Read the model definition and answer for the solid it produces. Units are mm, in the model's axes. A direction names the side the tool comes from. Coordinates: 2 decimals unless noted, no trailing zeros. Write each loop counter-clockwise with the first axis right and the second up, starting at its lowest first coordinate (ties: lowest second). Pieces come first, ordered by that corner, then holes. Notation, with made-up numbers: (86, 77.25) -> (132, 77.25) arc R29 ccw to (132, 101.25) -> close; hole circle Ø9 at (-40, -20.75). An arc over 180 degrees is marked (long way). Return JSON: item names as keys, results as strings.
from build123d import *

# Parameters (mm, degrees)
F1_W     = 740
F1_H     = 640
F1_W_2   = 20
F1_H_2   = 600
F2_DEPTH = 20
F0_R     = 1.4
F0_R_2   = 1.9
F0_W     = 5
F0_H     = 5
F0_R_3   = 16
F3_DEPTH = 5
F4_W     = 20
F4_H     = 20
F5_DEPTH = 700


with BuildPart() as f2:
    # F1 (on Top) → F2 (new body)
    with BuildSketch(Plane.XY):
        with Locations((0, -40)):
            Rectangle(F1_W, F1_H)
        Polygon((-350, -340), (-350, 260), (-147.5, 260), (-127.5, 260), (127.5, 260), (147.5, 260), (350, 260), (350, -340), (147.5, -340), (127.5, -340), (-127.5, -340), (-147.5, -340), align=None, mode=Mode.SUBTRACT)
        with Locations((137.5, -40)):
            Rectangle(F1_W_2, F1_H_2)
        with Locations((-137.5, -40)):
            Rectangle(F1_W_2, F1_H_2)
    extrude(amount=-F2_DEPTH)

    # F0 (on Top) → F3 (join)
    with BuildSketch(Plane.XY):
        with BuildLine():
            Line((330, -340), (-330, -340))
            Line((-330, -340), (-330, -379.616912))
            ThreePointArc((-330, -379.616912), (0, -503), (330, -379.616912))
            Line((330, -379.616912), (330, -340))
        make_face()
        with Locations((-285.202138, -385.913671)):
            Circle(F0_R, mode=Mode.SUBTRACT)
        with Locations((-313.348072, -363.468038)):
            Circle(F0_R, mode=Mode.SUBTRACT)
        with Locations((-124.358751, -463.371764)):
            Circle(F0_R, mode=Mode.SUBTRACT)
        with Locations((-89.261346, -471.382518)):
            Circle(F0_R, mode=Mode.SUBTRACT)
        with Locations((89.261346, -471.382518)):
            Circle(F0_R, mode=Mode.SUBTRACT)
        with Locations((124.358751, -463.371764)):
            Circle(F0_R, mode=Mode.SUBTRACT)
        with Locations((285.202138, -385.913671)):
            Circle(F0_R, mode=Mode.SUBTRACT)
        with Locations((313.348072, -363.468038)):
            Circle(F0_R, mode=Mode.SUBTRACT)
        with BuildLine():
            Line((330, 260), (330, 368.951685))
            Line((330, 368.951685), (330, 379.616912))
            ThreePointArc((330, 379.616912), (319.49595, 388.498826), (308.752952, 397.090185))
            Line((308.752952, 397.090185), (275.202138, 397.090185))
            Line((275.202138, 397.090185), (206.772293, 298.352508))
            ThreePointArc((206.772293, 298.352508), (146.302539, 332.21163), (80.5, 353.961509))
            Line((80.5, 353.961509), (79.396479, 349.085021))
            Line((79.396479, 349.085021), (77.189345, 339.331634))
            Line((77.189345, 339.331634), (70.567941, 310.071473))
            Line((70.567941, 310.071473), (68.360806, 300.318086))
            Line((68.360806, 300.318086), (67.03647, 294.465807))
            Line((67.03647, 294.465807), (-67.03647, 294.465807))
            Line((-67.03647, 294.465807), (-68.360806, 300.318086))
            Line((-68.360806, 300.318086), (-70.567941, 310.071473))
            Line((-70.567941, 310.071473), (-77.189345, 339.331634))
            Line((-77.189345, 339.331634), (-79.396479, 349.085021))
            Line((-79.396479, 349.085021), (-80.5, 353.961509))
            ThreePointArc((-80.5, 353.961509), (-146.302539, 332.21163), (-206.772293, 298.352508))
            Line((-206.772293, 298.352508), (-275.202138, 397.090185))
            Line((-275.202138, 397.090185), (-308.752952, 397.090185))
            ThreePointArc((-308.752952, 397.090185), (-319.49595, 388.498826), (-330, 379.616912))
            Line((-330, 379.616912), (-330, 260))
            Line((-330, 260), (330, 260))
        make_face()
        with Locations((-313.348072, 364.644552)):
            Circle(F0_R, mode=Mode.SUBTRACT)
        with Locations((-285.202138, 387.090185)):
            Circle(F0_R, mode=Mode.SUBTRACT)
        with Locations((313.348072, 364.644552)):
            Circle(F0_R, mode=Mode.SUBTRACT)
        with Locations((285.202138, 387.090185)):
            Circle(F0_R, mode=Mode.SUBTRACT)
        Polygon((77.189345, 339.331634), (79.396479, 349.085021), (74.519786, 350.188588), (72.312651, 340.435201), align=None)
        Polygon((-74.519786, 350.188588), (-79.396479, 349.085021), (-77.189345, 339.331634), (-72.312651, 340.435201), align=None)
        Polygon((68.360806, 300.318086), (70.567941, 310.071473), (65.691247, 311.17504), (63.484113, 301.421653), align=None)
        Polygon((-65.691247, 311.17504), (-70.567941, 310.071473), (-68.360806, 300.318086), (-63.484113, 301.421653), align=None)
        with BuildLine():
            Line((442.050902, 240), (350, 240))
            Line((350, 240), (350, -240))
            Line((350, -240), (442.050902, -240))
            ThreePointArc((442.050902, -240), (502.730809, -16.453988), (456.79808, 210.581372))
            Line((456.79808, 210.581372), (407.539006, 186.859452))
            Line((407.539006, 186.859452), (403.634053, 194.968172))
            Line((403.634053, 194.968172), (399.729099, 203.076892))
            Line((399.729099, 203.076892), (448.971082, 226.790581))
            ThreePointArc((448.971082, 226.790581), (445.559947, 233.420937), (442.050902, 240))
        make_face()
        with Locations((424.655149, -223.893378)):
            Circle(F0_R, mode=Mode.SUBTRACT)
        with Locations((440.274964, -191.458498)):
            Circle(F0_R, mode=Mode.SUBTRACT)
        with Locations((480, -17.411743)):
            Circle(F0_R, mode=Mode.SUBTRACT)
        with Locations((480, 18.588257)):
            Circle(F0_R, mode=Mode.SUBTRACT)
        with Locations((419.869226, 188.912666)):
            Circle(F0_R_2, mode=Mode.SUBTRACT)
        with Locations((409.022132, 211.436888)):
            Circle(F0_R_2, mode=Mode.SUBTRACT)
        with BuildLine():
            Line((-350, -240), (-350, 240))
            Line((-350, 240), (-442.050902, 240))
            ThreePointArc((-442.050902, 240), (-503, 0), (-442.050902, -240))
            Line((-442.050902, -240), (-350, -240))
        make_face()
        with Locations((-424.655149, -223.893378)):
            Circle(F0_R, mode=Mode.SUBTRACT)
        with Locations((-440.274964, -191.458498)):
            Circle(F0_R, mode=Mode.SUBTRACT)
        with Locations((-480, -17.411743)):
            Circle(F0_R, mode=Mode.SUBTRACT)
        with Locations((-480, 18.588257)):
            Circle(F0_R, mode=Mode.SUBTRACT)
        with Locations((-440.274964, 192.635012)):
            Circle(F0_R, mode=Mode.SUBTRACT)
        with Locations((-424.655149, 225.069891)):
            Circle(F0_R, mode=Mode.SUBTRACT)
        with BuildLine():
            Line((-140, 130), (-150, 130))
            Line((-150, 130), (-150, -130))
            Line((-150, -130), (-140, -130))
            Line((-140, -130), (-140, -120))
            ThreePointArc((-140, -120), (-137.5, -117.5), (-135, -120))
            Line((-135, -120), (-134.791644, -130))
            Line((-134.791644, -130), (135, -130))
            Line((135, -130), (135, -120))
            ThreePointArc((135, -120), (137.5, -117.5), (140, -120))
            Line((140, -120), (140, -130))
            Line((140, -130), (150, -130))
            Line((150, -130), (150, 130))
            Line((150, 130), (140, 130))
            Line((140, 130), (140, 120))
            ThreePointArc((140, 120), (137.5, 117.5), (135, 120))
            Line((135, 120), (135, 130))
            Line((135, 130), (-135, 130))
            Line((-135, 130), (-135, 120))
            ThreePointArc((-135, 120), (-137.5, 117.5), (-140, 120))
            Line((-140, 120), (-140, 130))
        make_face()
        with Locations((-93.691649, -118.440386)):
            Circle(F0_R, mode=Mode.SUBTRACT)
        with Locations((-118.440386, -93.691649)):
            Circle(F0_R, mode=Mode.SUBTRACT)
        with Locations((93.691649, -118.440386)):
            Circle(F0_R, mode=Mode.SUBTRACT)
        with Locations((118.440386, -93.691649)):
            Circle(F0_R, mode=Mode.SUBTRACT)
        with Locations((-12.5, -19.5)):
            Rectangle(F0_W, F0_H, mode=Mode.SUBTRACT)
        Circle(F0_R_3, mode=Mode.SUBTRACT)
        with Locations((-12.5, 19.5)):
            Rectangle(F0_W, F0_H, mode=Mode.SUBTRACT)
        with Locations((-118.440386, 93.691649)):
            Circle(F0_R, mode=Mode.SUBTRACT)
        with Locations((-93.691649, 118.440386)):
            Circle(F0_R, mode=Mode.SUBTRACT)
        with Locations((12.5, -19.5)):
            Rectangle(F0_W, F0_H, mode=Mode.SUBTRACT)
        with Locations((12.5, 19.5)):
            Rectangle(F0_W, F0_H, mode=Mode.SUBTRACT)
        with Locations((118.440386, 93.691649)):
            Circle(F0_R, mode=Mode.SUBTRACT)
        with Locations((93.691649, 118.440386)):
            Circle(F0_R, mode=Mode.SUBTRACT)
    extrude(amount=F3_DEPTH)

    # F4 (on face) → F5 (join)
    with BuildSketch(Plane(origin=(0, 0, -20), x_dir=(1, 0, 0), z_dir=(0, 0, -1))):
        with Locations((-340, 350)):
            Rectangle(F4_W, F4_H)
        with Locations((340, 350)):
            Rectangle(F4_W, F4_H)
        with Locations((-340, -270)):
            Rectangle(F4_W, F4_H)
        with Locations((340, -270)):
            Rectangle(F4_W, F4_H)
    extrude(amount=F5_DEPTH)


solid = f2.part
1. A tool of negligible diameter and unlimited length cuts with its end or side. For faces 1 (the face through (-359, -299, 0)), 2 (the face through (-331, -360, -198)), 3 (the face through (241.466, 348.413, 2.465)), from which of +Z, -Z, +X, -X, +Y, -Y can it reach the whole face along a straight path? Write none if from no direction.
Taken from the geometry:
{"face 1": "+Z, -X, -Y", "face 2": "-Z, +X, -X, -Y", "face 3": "+Z, -Z, +Y"}
2. The part is cut by section B-B (y = 64.5). Determine the outline of the cut face in (x, z).
Taken from the geometry:
{"outline": "(-498.85, 0) -> (-370, 0) -> (-370, -20) -> (-350, -20) -> (-350, 5) -> (-498.85, 5) -> close; (-150, 0) -> (-147.5, 0) -> (-147.5, -20) -> (-127.5, -20) -> (-127.5, 0) -> (127.5, 0) -> (127.5, -20) -> (147.5, -20) -> (147.5, 0) -> (150, 0) -> (150, 5) -> (-150, 5) -> close; (350, -20) -> (370, -20) -> (370, 0) -> (498.85, 0) -> (498.85, 5) -> (350, 5) -> close"}
3. Flat-ended cylindrical pins translate along their axes: pin 1 Ø5.5 at (y, z) = (-127, 1.5) entering from -X; pin 2 Ø4.5 at (x, y) = (-313.35, 364.64) entering from +Z; pin 3 Ø2.5 at (x, z) = (396, 2) entering from +Y; pin 4 Ø4.5 at (x, y) = (118.44, -93.69) entering from -Z. Find the tip coordinate at first contact, or state that the pin passes through.
Taken from the geometry:
{"pin 1": "stops at x = -487.41", "pin 2": "stops at z = 5", "pin 3": "stops at y = 240", "pin 4": "stops at z = 0"}
4. For a pull along Y with two mould halves and no side action, classify faces 4 (the face through (-30, 2, 0)), 5 (the face through (354, 265, 0)), 6 (the face through (-331, 280, -198)), 7 (the face through (432.513, 198.886, 2.465)) as +Y half, -Y half, draft (parallel to the pull), parting line (faces both ways), or undercut.
Taken from the geometry:
{"face 4": "undercut", "face 5": "draft", "face 6": "+Y half", "face 7": "undercut"}
5. The part is cut by section C-C (y = -63.5). Determine the outline of the cut face in (x, z).
Taken from the geometry:
{"outline": "(-498.98, 0) -> (-370, 0) -> (-370, -20) -> (-350, -20) -> (-350, 5) -> (-498.98, 5) -> close; (-150, 0) -> (-147.5, 0) -> (-147.5, -20) -> (-127.5, -20) -> (-127.5, 0) -> (127.5, 0) -> (127.5, -20) -> (147.5, -20) -> (147.5, 0) -> (150, 0) -> (150, 5) -> (-150, 5) -> close; (350, -20) -> (370, -20) -> (370, 0) -> (498.98, 0) -> (498.98, 5) -> (350, 5) -> close"}
6. Consider L1, parallel to X at y = -351, z = -478; L2, parallel to Y at x = -339.5, z = -351.5; L3, parallel to Z at x = 405.5, y = -60. Determine where each line is inside the solid, lowest interval first.
Taken from the geometry:
{"L1": "x = -350 to -330, 330 to 350", "L2": "y = -360 to -340, 260 to 280", "L3": "z = 0 to 5"}
7. The part is cut by section A-A (z = -422.5). Determine the outline of the cut face in (x, y), then the cut area to 3 significant figures.
Taken from the geometry:
{"outline": "(-350, -360) -> (-330, -360) -> (-330, -340) -> (-350, -340) -> close; (-350, 260) -> (-330, 260) -> (-330, 280) -> (-350, 280) -> close; (330, -360) -> (350, -360) -> (350, -340) -> (330, -340) -> close; (330, 260) -> (350, 260) -> (350, 280) -> (330, 280) -> close", "area": "1,600 mm2"}
